The figure shows three views and two pictorial views of one solid part (mm, origin at its lowest corner). Answer the questions. A direction names the side the tool comes from. Give positions to 0.01 mm unless a question says otherwise; leave off trailing zeros. Write each loop counter-clockwise with the first axis right and the second up, starting at its lowest first coordinate (ties: lowest second). Pieces come first, ordered by that corner, then holes. Notation, with made-up numbers: (-24.5, 77.5) -> (-1.5, 77.5) arc R25 ccw to (-1.5, 90.5) -> close; hole circle Ø6 at (40.5, -34.75). An arc over 180 degrees is marked (long way). Use a Markdown table: item, result.
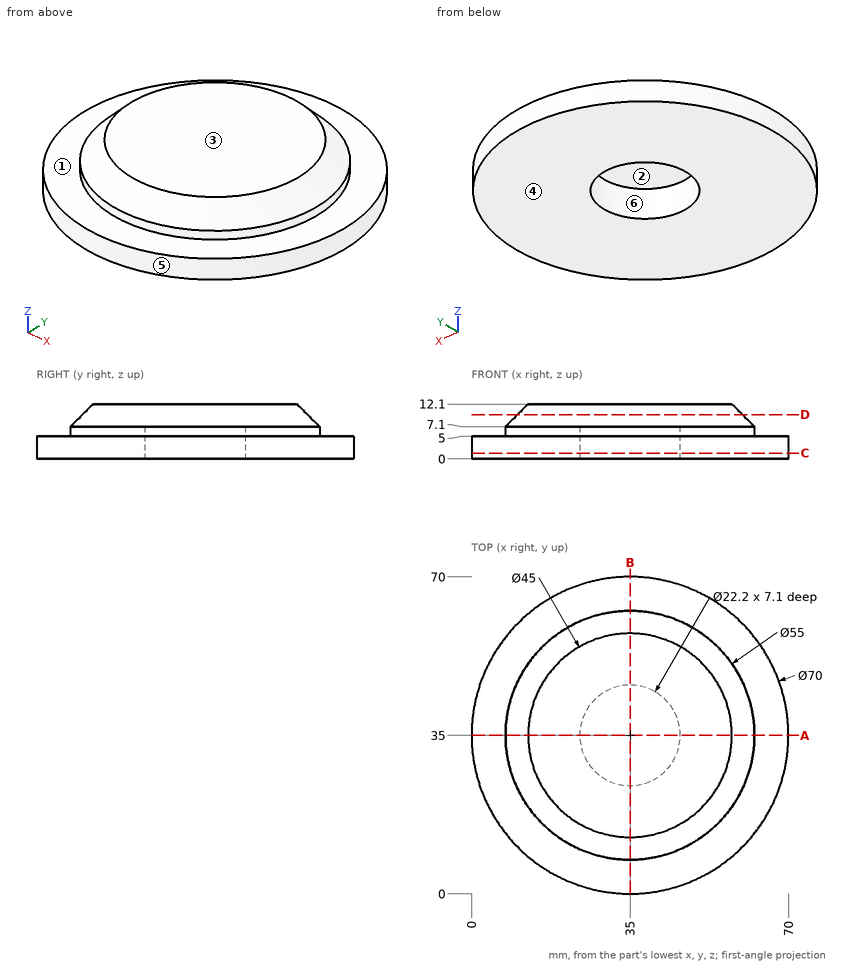
Item 1: A cutting plane is placed at D-D (z = 9.75). Give the vertices of the cut face in (x, y), then the cut area to 3 significant figures.
Return value:
| item | result |
|---|---|
| outline | circle Ø49.7 at (35, 35) |
| area | 1,940 mm^2 |
Item 2: A cutting plane is placed at C-C (z = 1.25). Give the vertices of the cut face in (x, y), then the cut area to 3 significant figures.
Return value:
| item | result |
|---|---|
| outline | circle Ø70 at (35, 35); hole circle Ø22.2 at (35, 35) |
| area | 3,460 mm^2 |
Item 3: A tool of negligible diameter and unlimited length cuts with its end or side. For the marked faces 1, 2 and 3, from which of +Z, -Z, +X, -X, +Y, -Y can it reach the whole face along a straight path? Write none if from no direction.
Return value:
| item | result |
|---|---|
| face 1 | +Z |
| face 2 | -Z |
| face 3 | +Z, +X, -X, +Y, -Y |
Item 4: For a pull along Y with two mould halves and no side action, classify the marked faces 4, 5 and 6 as +Y half, -Y half, draft (parallel to the pull), parting line (faces both ways), or undercut.
Return value:
| item | result |
|---|---|
| face 4 | draft |
| face 5 | parting line |
| face 6 | undercut |
Item 5: Each of these flat-tipped pins is pushed along its axis until it touches: P1, Ø2, axis at x = 24, z = 7, coming from the -Y side; P2, Ø12, axis at x = 14.5, y = 58.5, coming from the -Z side; P3, Ø6, axis at x = 44, z = 6, coming from the +Y side; P4, Ø1.5, axis at y = 24, z = 9.5, coming from the -X side. Where does it stop, or does it pass through?
Return value:
| item | result |
|---|---|
| P1 | y = 9.38 |
| P2 | z = 0 |
| P3 | y = 69.45 |
| P4 | x = 11.54 |
Item 6: A cutting plane is placed at A-A (y = 35). Give the vertices of the cut face in (x, z).
Return value:
| item | result |
|---|---|
| outline | (0, 0) -> (23.9, 0) -> (23.9, 7.1) -> (46.1, 7.1) -> (46.1, 0) -> (70, 0) -> (70, 5) -> (62.5, 5) -> (62.5, 7.1) -> (57.5, 12.1) -> (12.5, 12.1) -> (7.5, 7.1) -> (7.5, 5) -> (0, 5) -> close |
Item 7: Straight lines are drawn through the part: line 1 along Y through (x, z) = (35, 4.75); line 2 along Y through (x, z) = (44, 0.75); line 3 along Z through (x, y) = (29, 67.5). For each, find the intervals that lie inside material, in ascending order. Write a range as [from, to].
Return value:
| item | result |
|---|---|
| line 1 | [0, 23.9], [46.1, 70] |
| line 2 | [1.18, 28.5], [41.5, 68.82] |
| line 3 | [0, 5] |
